from build123d import *

# Parameters (mm, degrees)
SKETCH_1_R      = 2
EXTRUDE_1_DEPTH = 2
FILLET_1_R      = 2


with BuildPart() as part:
    # 草图1 → 凸台-拉伸1 (new body)
    with BuildSketch(Plane.XY):
        with BuildLine():
            Line((-42.723571429, 9.145714286), (-42.723571429, 22.145714286))
            Line((-42.723571429, 22.145714286), (-54.723571429, 22.145714286))
            Line((-54.723571429, 22.145714286), (-54.723571429, -21.854285714))
            Line((-54.723571429, -21.854285714), (-42.723571429, -21.854285714))
            Line((-42.723571429, -21.854285714), (-42.723571429, -8.854285714))
            Line((-42.723571429, -8.854285714), (28.047672016, -8.854285714))
            ThreePointArc((28.047672016, -8.854285714), (57.276428571, 0.145714286), (28.047672016, 9.145714286))
            Line((28.047672016, 9.145714286), (-42.723571429, 9.145714286))
        make_face()
        with Locations((1.276428571, 0.145714286)):
            Circle(SKETCH_1_R, mode=Mode.SUBTRACT)
        with Locations((-48.723571429, 16.645714286)):
            Circle(SKETCH_1_R, mode=Mode.SUBTRACT)
        with Locations((-48.723571429, -16.354285714)):
            Circle(SKETCH_1_R, mode=Mode.SUBTRACT)
        with Locations((49.776428571, -8.354285714)):
            Circle(SKETCH_1_R, mode=Mode.SUBTRACT)
        with Locations((32.776428571, -8.354285714)):
            Circle(SKETCH_1_R, mode=Mode.SUBTRACT)
        with Locations((32.776428571, 8.645714286)):
            Circle(SKETCH_1_R, mode=Mode.SUBTRACT)
        with Locations((49.776428571, 8.645714286)):
            Circle(SKETCH_1_R, mode=Mode.SUBTRACT)
    extrude(amount=EXTRUDE_1_DEPTH)

    # 圆角1
    fillet_1_edges = [part.edges().sort_by_distance(p)[0] for p in [
        (-42.723571429, -21.854285714, 1),
        (-54.723571429, -21.854285714, 1),
        (-54.723571429, 22.145714286, 1),
        (-42.723571429, 22.145714286, 1),
    ]]
    fillet(fillet_1_edges, radius=FILLET_1_R)


solid = part.part
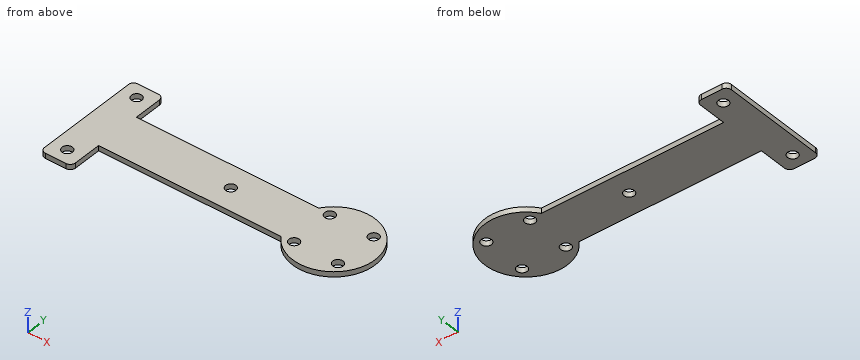
The listing builds one solid part. Answer for the finished solid, in the listing's coordinates (mm). Coordinates: 2 decimals unless noted, no trailing zeros. Write each loop counter-clockwise with the first axis right and the second up, starting at its lowest first coordinate (ties: lowest second). Pieces come first, ordered by that corner, then holes. Notation, with made-up numbers: (-36.75, -1.5) - (-32.75, -1.5) arc R18 ccw to (-32.75, 25.5) - close; hole circle Ø3 at (-19.75, 62). An arc over 180 degrees is marked (long way). Answer as CSV lines item,"result".
1. Given P1, Ø4.5, axis at x = 49.78, y = -8.35, coming from the -Z side; P2, Ø3, axis at x = -48.72, y = -16.35, coming from the +Z side; P3, Ø0.6, axis at x = -0.5, z = 0.5, coming from the -Y side, each flat-ended and moving along its own axis, determine where each tip first touches the part or whether it passes through.
Computed values:
P1,"stops at z = 0"
P2,"passes through"
P3,"stops at y = -8.85"
2. Straight lines are drawn through the part: line 1 (X direction, y = 8, z = 1.5); line 2 (Y direction, x = -2, z = 0.6); line 3 (Y direction, x = 41, z = 1.8). For each, find the intervals that lie inside material, in ascending order. Write a range as [from, to].
Computed values:
line 1,"x = [-54.72, 30.88], [34.67, 47.88], [51.67, 55.22]"
line 2,"y = [-8.85, 9.15]"
line 3,"y = [-15.85, 16.14]"
3. Find section A-A (z = 1.15). Give the vertices of the cut face in (x, y).
Computed values:
outline,"(-54.72, -19.85) arc R2 ccw to (-52.72, -21.85) - (-44.72, -21.85) arc R2 ccw to (-42.72, -19.85) - (-42.72, -8.85) - (28.05, -8.85) arc R16 ccw (long way) to (28.05, 9.15) - (-42.72, 9.15) - (-42.72, 20.15) arc R2 ccw to (-44.72, 22.15) - (-52.72, 22.15) arc R2 ccw to (-54.72, 20.15) - close; hole circle Ø4 at (-48.72, -16.35); hole circle Ø4 at (-48.72, 16.65); hole circle Ø4 at (1.28, 0.15); hole circle Ø4 at (32.78, -8.35); hole circle Ø4 at (32.78, 8.65); hole circle Ø4 at (49.78, -8.35); hole circle Ø4 at (49.78, 8.65)"
4. Find section C-C (x = -21). Give the vertices of the cut face in (y, z), plus the area to 3 significant figures.
Computed values:
outline,"(-8.85, 0) - (9.15, 0) - (9.15, 2) - (-8.85, 2) - close"
area,"36.0 mm²"
5. Find section B-B (y = -11.5). Give the vertices of the cut face in (x, z), plus the area to 3 significant figures.
Computed values:
outline,"(-54.72, 0) - (-42.72, 0) - (-42.72, 2) - (-54.72, 2) - close; (30.3, 0) - (52.25, 0) - (52.25, 2) - (30.3, 2) - close"
area,"67.9 mm²"
